from build123d import *

# Parameters (mm, degrees)
CYLINDER036_R      = 3.5
CYLINDER036_DEPTH  = 4.75
CYLINDER035_R      = 2
CYLINDER035_DEPTH  = 18
CYLINDER033_R      = 4
CYLINDER033_DEPTH  = 14
BOX012_W           = 1
BOX012_H           = 10
BOX012_DEPTH       = 14
CYLINDER034_R      = 2.75
CYLINDER034_DEPTH  = 6
CYLINDER032_R      = 2.75
CYLINDER032_DEPTH  = 6
BOX011_W           = 42
BOX011_H           = 6
BOX011_DEPTH       = 14
BOX013_W           = 18
BOX013_H           = 27
BOX013_DEPTH       = 14
CHAMFER001005_SIZE = 0.5
CHAMFER001003_SIZE = 0.2


with BuildPart() as cylinder036:
    # Cylinder036 → Cylinder036 (new body)
    with BuildSketch(Plane(origin=(0, 21.75, 7), x_dir=(0, 0, -1), z_dir=(1, 0, 0))):
        Circle(CYLINDER036_R)
    extrude(amount=CYLINDER036_DEPTH)


with BuildPart() as cylinder035:
    # Cylinder035 → Cylinder035 (new body)
    with BuildSketch(Plane(origin=(0, 21.75, 7), x_dir=(0, 0, -1), z_dir=(1, 0, 0))):
        Circle(CYLINDER035_R)
    extrude(amount=CYLINDER035_DEPTH)


with BuildPart() as cylinder033:
    # Cylinder033 → Cylinder033 (new body)
    with BuildSketch(Plane(origin=(9, 14, 0), x_dir=(1, 0, 0), z_dir=(0, 0, 1))):
        Circle(CYLINDER033_R)
    extrude(amount=CYLINDER033_DEPTH)


with BuildPart() as cube007:
    # Box012 → Box012 (new body)
    with BuildSketch(Plane(origin=(8.5, 17, 0), x_dir=(1, 0, 0), z_dir=(0, 0, 1))):
        with Locations((0.5, 5)):
            Rectangle(BOX012_W, BOX012_H)
    extrude(amount=BOX012_DEPTH)


with BuildPart() as cylinder034:
    # Cylinder034 → Cylinder034 (new body)
    with BuildSketch(Plane(origin=(24.75, 0, 7), x_dir=(1, 0, 0), z_dir=(0, -1, 0))):
        Circle(CYLINDER034_R)
    extrude(amount=CYLINDER034_DEPTH)


with BuildPart() as cylinder032:
    # Cylinder032 → Cylinder032 (new body)
    with BuildSketch(Plane(origin=(-6.75, 0, 7), x_dir=(1, 0, 0), z_dir=(0, -1, 0))):
        Circle(CYLINDER032_R)
    extrude(amount=CYLINDER032_DEPTH)


with BuildPart() as cube006:
    # Box011 → Box011 (new body)
    with BuildSketch(Plane(origin=(-12, -6, 0), x_dir=(1, 0, 0), z_dir=(0, 0, 1))):
        with Locations((21, 3)):
            Rectangle(BOX011_W, BOX011_H)
    extrude(amount=BOX011_DEPTH)


with BuildPart() as chamfer001003:
    # Box013 → Box013 (new body)
    with BuildSketch(Plane.XY):
        with Locations((9, 13.5)):
            Rectangle(BOX013_W, BOX013_H)
    extrude(amount=BOX013_DEPTH)

    # Fusion007005: union Cube006
    add(cube006.part)

    # Cut002021: cut Cylinder032
    add(cylinder032.part, mode=Mode.SUBTRACT)

    # Cut002017: cut Cylinder034
    add(cylinder034.part, mode=Mode.SUBTRACT)

    # Cut002022: cut Cube007
    add(cube007.part, mode=Mode.SUBTRACT)

    # Cut002018: cut Cylinder033
    add(cylinder033.part, mode=Mode.SUBTRACT)

    # Cut002019: cut Cylinder035
    add(cylinder035.part, mode=Mode.SUBTRACT)

    # Cut002020: cut Cylinder036
    add(cylinder036.part, mode=Mode.SUBTRACT)

    # Chamfer001005
    chamfer001005_edges = [chamfer001003.edges().sort_by_distance(p)[0] for p in [
        (0, 21.75, 10.5),
        (-9.5, 0, 7),
        (22, 0, 7),
        (-9.5, -6, 7),
        (22, -6, 7),
    ]]
    chamfer(chamfer001005_edges, length=CHAMFER001005_SIZE)

    # Chamfer001003
    chamfer001003_edges = [chamfer001003.edges().sort_by_distance(p)[0] for p in [
        (6.354249, 11, 14),
        (12, 16.645751, 14),
        (6.354249, 11, 0),
        (12, 16.645751, 0),
        (18, 21.75, 9),
    ]]
    chamfer(chamfer001003_edges, length=CHAMFER001003_SIZE)


solid = chamfer001003.part
Verification items for the finished model (mm, model axes). A direction names the side the tool comes from. Give positions to 0.01 mm unless a question says otherwise; leave off trailing zeros. Order: outer loops, then holes, each group sorted by start corner. A loop starts at its lowest first (then second) coordinate and runs counter-clockwise, first axis right, second up. Notation, with made-up numbers: M 9,50.25 L 18,50.25 A14 cw 18,75.25 Z; hole C 35.5,78 d7. An arc over 180 degrees is marked long. Use one line per item in the form item = value. Start each with the question number.
Q1. Section check A-A (y = 21.75). Enter the section's corners in (x, z).
Q2. Go/stop test with flat-tipped pins: pin 1 Ø7 at (x, z) = (24.75, 7) entering from +Y; pin 2 Ø4 at (y, z) = (10.5, 4.5) entering from -X; pin 3 Ø7 at (y, z) = (20.5, 4) entering from +X. Record where each tip stops, or that it passes through.
Q3. Section check D-D (z = 1.5). Enter the section's corners in (x, y).
Q4. Mould release check, pull along Y, two halves, no side actions. Record for faces 4 (the flat face through (18, 13, 7)), 5 (the flat face through (-3, 0, 7)), 6 (the cylindrical face through (13.6, 21.8, 9)): +Y half, -Y half, draft (parallel to the pull), parting line (faces both ways), or undercut.
Q5. Section check C-C (y = 14). Enter the section's corners in (x, z).
Q6. Access from +Z, -Z, +X, -X, +Y, -Y to the whole of each face (thin tool, end or side, straight path). Record for faces 1 (the flat face through (0, 10, 7)), 2 (the cylindrical face through (2.6, 25.22, 7.46)), 3 (the cylindrical face through (6.6, 21.8, 9)).
Q7. Section check B-B (x = -6.75). Enter the section's corners in (y, z).
Q8. Scan lines: line 1 along Y through (x, z) = (7.6, 7); line 2 along Z through (x, y) = (-6.75, -3); line 3 along X through (y, z) = (14, 7.5). Record each from-to range of solid material in increasing order. Write a range as [from, to].
Evaluation:
q1.outline = M 0,0 L 8.5,0 L 8.5,5 L 4.75,5 L 4.75,3.5 L 0.5,3.5 L 0,3 Z; M 0,11 L 0.5,10.5 L 4.75,10.5 L 4.75,9 L 8.5,9 L 8.5,14 L 0,14 Z; M 9.5,0 L 18,0 L 18,4.8 L 17.8,5 L 9.5,5 Z; M 9.5,9 L 17.8,9 L 18,9.2 L 18,14 L 9.5,14 Z
q2.pin_1 = 0
q2.pin_2 = 0
q2.pin_3 = 18
q3.outline = M -12,-6 L 30,-6 L 30,0 L 18,0 L 18,27 L 9.5,27 L 9.5,17.97 A4 cw long 8.5,17.97 L 8.5,27 L 0,27 L 0,0 L -12,0 Z
q4.face_4 = draft
q4.face_5 = +Y half
q4.face_6 = undercut
q5.outline = M 0,0 L 4.8,0 L 5,0.2 L 5,13.8 L 4.8,14 L 0,14 Z; M 13,0.2 L 13.2,0 L 18,0 L 18,14 L 13.2,14 L 13,13.8 Z
q6.face_1 = +Z, -Z, -X, +Y
q6.face_2 = -X
q6.face_3 = +X, -X
q7.outline = M -6,0 L 0,0 L 0,3.75 L -0.5,4.25 L -5.5,4.25 L -6,3.75 Z; M -6,10.25 L -5.5,9.75 L -0.5,9.75 L 0,10.25 L 0,14 L -6,14 Z
q8.line_1 = [-6, 10.25], [17.75, 19.75], [23.75, 27]
q8.line_2 = [0, 4.25], [9.75, 14]
q8.line_3 = [0, 5], [13, 18]
